The figure shows three views and two pictorial views of one solid part (mm, origin at its lowest corner). Answer the questions. A direction names the side the tool comes from. Give positions to 0.01 mm unless a question says otherwise; leave off trailing zeros. Order: outer loops, then holes, each group sorted by start corner. A loop starts at its lowest first (then second) coordinate and runs counter-clockwise, first axis right, second up. Notation, with made-up numbers: (-8, 19.25) - (0, 19.25) arc R5 cw to (0, 25.25) - close; hole circle Ø4 at (15, 41). An arc over 180 degrees is marked (long way). Answer as CSV lines item,"result". Start each with the question number.
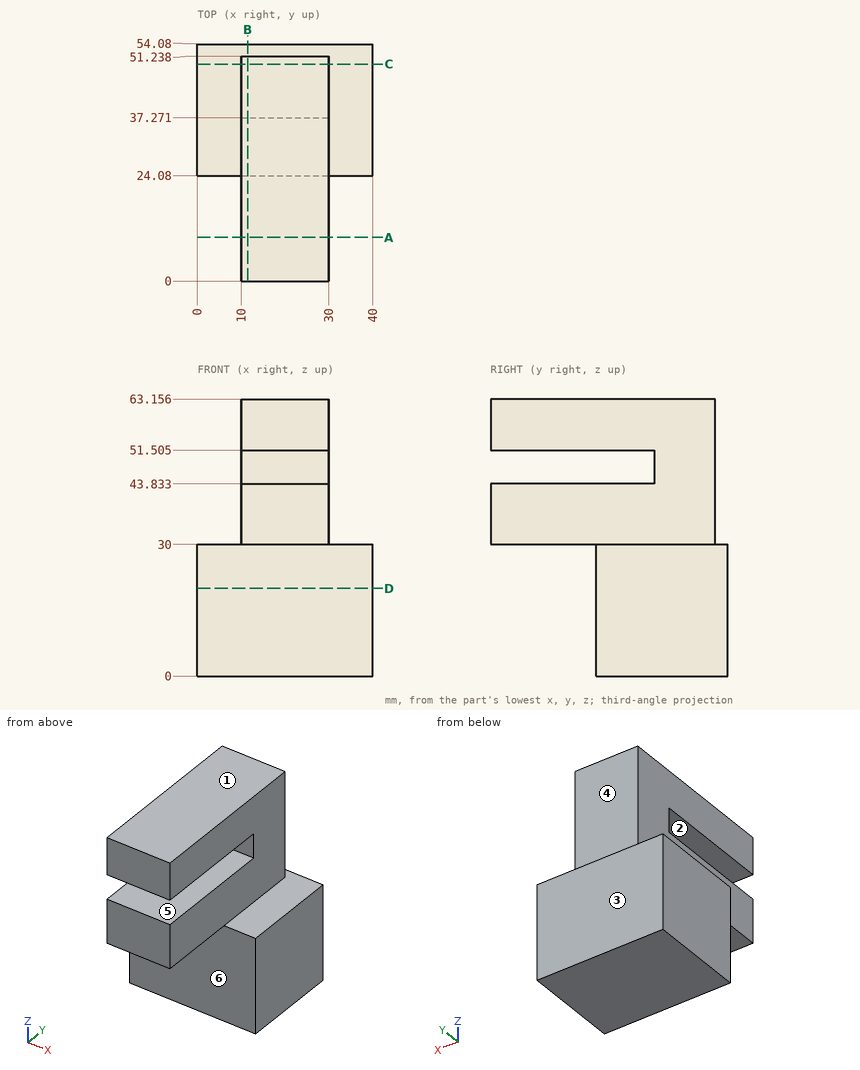
(1) Determine the mould class of the marked faces 1, 2 and 3 for opening direction Z: released by +Z, released by -Z, zero draft, split by the parting line, or undercut.
(2) Straight lines are drawn through the part: line 1 (Z direction, x = 12.5, y = 18.5) (1 decimal); line 2 (Z direction, x = 16.5, y = 31) (1 decimal); line 3 (Y direction, x = 13.5, z = 52). For each, find the intervals that lie inside material, in ascending order. Write a range as [from, to].
(3) Section C-C, the plane y = 49.5 is taken. Write down the section's boundary in (x, z).
(4) Section D-D, the plane z = 20 is taken. Write down the section's boundary in (x, y).
(5) Flat-ended cylindrical pins translate along their axes: pin 1 Ø1 at (y, z) = (48.5, 42) entering from -X; pin 2 Ø22 at (x, y) = (15.5, 16.5) entering from -Z; pin 3 Ø9 at (x, z) = (22, 11) entering from -Y; pin 4 Ø22 at (x, y) = (19, 6.5) entering from -Z. Find the tip coordinate at first contact, or state that the pin passes through.
(6) Section B-B, the plane x = 11.5 is taken. Write down the section's boundary in (y, z) (1 decimal).
(7) Section A-A, the plane y = 10 is taken. Write down the section's boundary in (x, z) (1 decimal), and give its area (3 significant figures).
(8) Which of the six approach directions +Z, -Z, +X, -X, +Y, -Y give full straight-line access (tool end or side, diameter ignored) to the marked faces 4, 5 and 6?
Checks:
1,face 1,"released by +Z"
1,face 2,"undercut"
1,face 3,"zero draft"
2,line 1,"z = [30, 43.8], [51.5, 63.2]"
2,line 2,"z = [0, 43.8], [51.5, 63.2]"
2,line 3,"y = [0, 51.24]"
3,outline,"(0, 0) - (40, 0) - (40, 30) - (30, 30) - (30, 63.16) - (10, 63.16) - (10, 30) - (0, 30) - close"
4,outline,"(0, 24.08) - (40, 24.08) - (40, 54.08) - (0, 54.08) - close"
5,pin 1,"stops at x = 10"
5,pin 2,"stops at z = 0"
5,pin 3,"stops at y = 24.08"
5,pin 4,"stops at z = 30"
6,outline,"(0, 30) - (24.1, 30) - (24.1, 0) - (54.1, 0) - (54.1, 30) - (51.2, 30) - (51.2, 63.2) - (0, 63.2) - (0, 51.5) - (37.3, 51.5) - (37.3, 43.8) - (0, 43.8) - close"
7,outline,"(10, 30) - (30, 30) - (30, 43.8) - (10, 43.8) - close; (10, 51.5) - (30, 51.5) - (30, 63.2) - (10, 63.2) - close"
7,area,"510 mm²"
8,face 4,"+Z, +X, -X, +Y"
8,face 5,"+X, -X, -Y"
8,face 6,"-Z, +X, -X, -Y"
